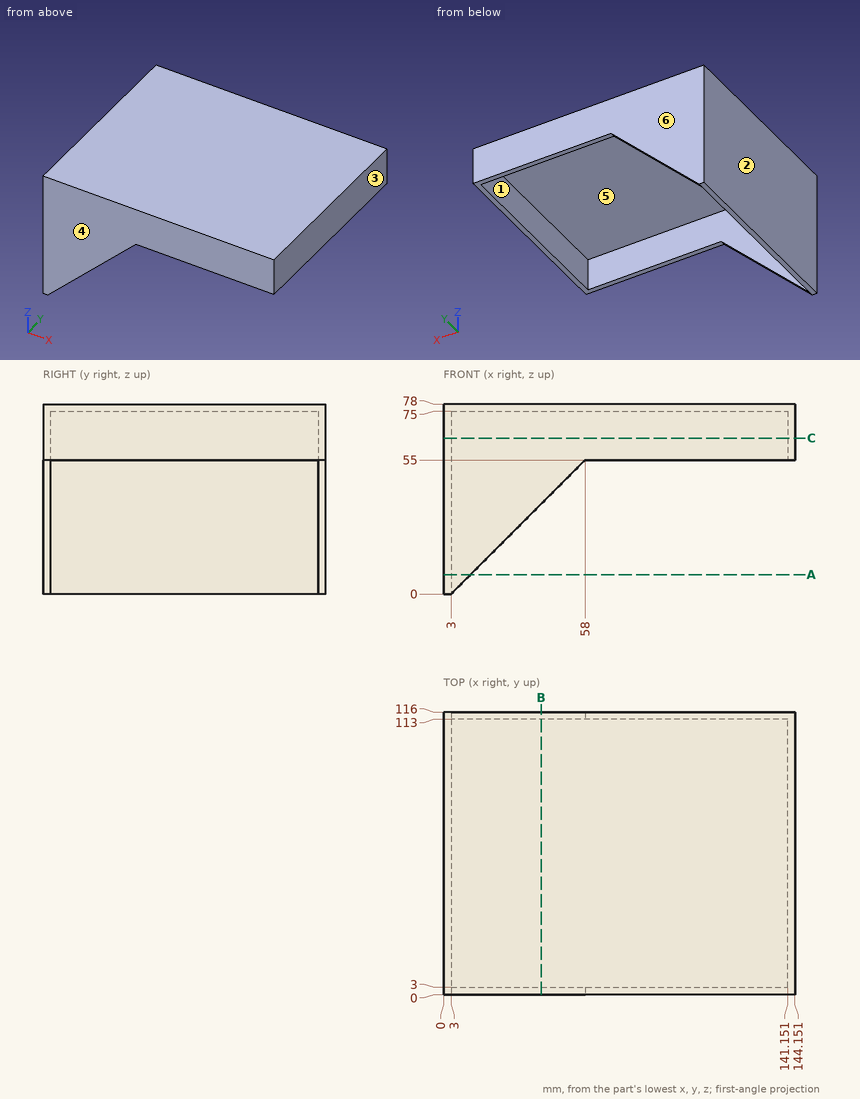
The figure shows three views and two pictorial views of one solid part (mm, origin at its lowest corner). Answer the questions. A direction names the side the tool comes from. Give positions to 0.01 mm unless a question says otherwise; leave off trailing zeros. Write each loop counter-clockwise with the first axis right and the second up, starting at its lowest first coordinate (ties: lowest second). Pieces come first, ordered by that corner, then holes. Notation, with made-up numbers: (53.25, 24) - (64.25, 24) arc R21 ccw to (64.25, 59) - close; hole circle Ø1 at (-34.75, 51). An arc over 180 degrees is marked (long way). Use one line per item in the form item = value. Start each with the question number.
1) Consider line 1 along X through (y, z) = (9.5, 73); line 2 along Y through (x, z) = (54, 58.5); line 3 along Z through (x, y) = (64, 63). Determine where each line is inside the solid, lowest interval first. Write a range as from..to.
2) Flat-ended cylindrical pins translate along their axes: pin 1 Ø2 at (x, y) = (78, 69) entering from -Z; pin 2 Ø8 at (y, z) = (35.5, 35) entering from +X. Find the tip coordinate at first contact, or state that the pin passes through.
3) Find section A-A on z = 8. Determine the outline of the cut face in (x, y).
4) Find section B-B on x = 40. Determine the outline of the cut face in (y, z).
5) Find section C-C on z = 64. Determine the outline of the cut face in (x, y).
6) A tool of negligible diameter and unlimited length cuts with its end or side. For the marked faces 5 and 6, from which of +Z, -Z, +X, -X, +Y, -Y can it reach the whole face along a straight path? Write none if from no direction.
7) The mould has two halves that part along X. Classify the marked faces 1, 2, 3 and 4: pulls with the +X half, pulls with the -X half, needs draft (parallel to the pull), parting line crosses it, or undercut.
Geometry results:
q1.line_1 = 0..3, 141.15..144.15
q1.line_2 = 0..3, 113..116
q1.line_3 = 75..78
q2.pin_1 = 75
q2.pin_2 = 3
q3.outline = (0, 0) - (11, 0) - (11, 3) - (3, 3) - (3, 113) - (11, 113) - (11, 116) - (0, 116) - close
q4.outline = (0, 37) - (3, 37) - (3, 75) - (113, 75) - (113, 37) - (116, 37) - (116, 78) - (0, 78) - close
q5.outline = (0, 0) - (144.15, 0) - (144.15, 116) - (0, 116) - close; hole (3, 3) - (141.15, 3) - (141.15, 113) - (3, 113) - close
q6.face_5 = -Z
q6.face_6 = +Z, -Z, +X, -X, +Y
q7.face_1 = undercut
q7.face_2 = pulls with the -X half
q7.face_3 = pulls with the +X half
q7.face_4 = needs draft
